Input: dimensioned drawing with shaded views. Units: mm. Origin: part minimum x, y, z. A direction names the side the tool comes from. Round coordinates to 2 decimals unless told otherwise and drop trailing zeros. Loops run counter-clockwise (first coordinate to the right, second up) from the corner with the lowest first, then second, coordinate; pieces in that order, holes last. Notation, with made-up numbers: (-4.75, 58) - (8.25, 58) arc R14 cw to (8.25, 74) - close; hole circle Ø6 at (-11.75, 54). An arc over 180 degrees is marked (long way). Answer as CSV lines item,"result".
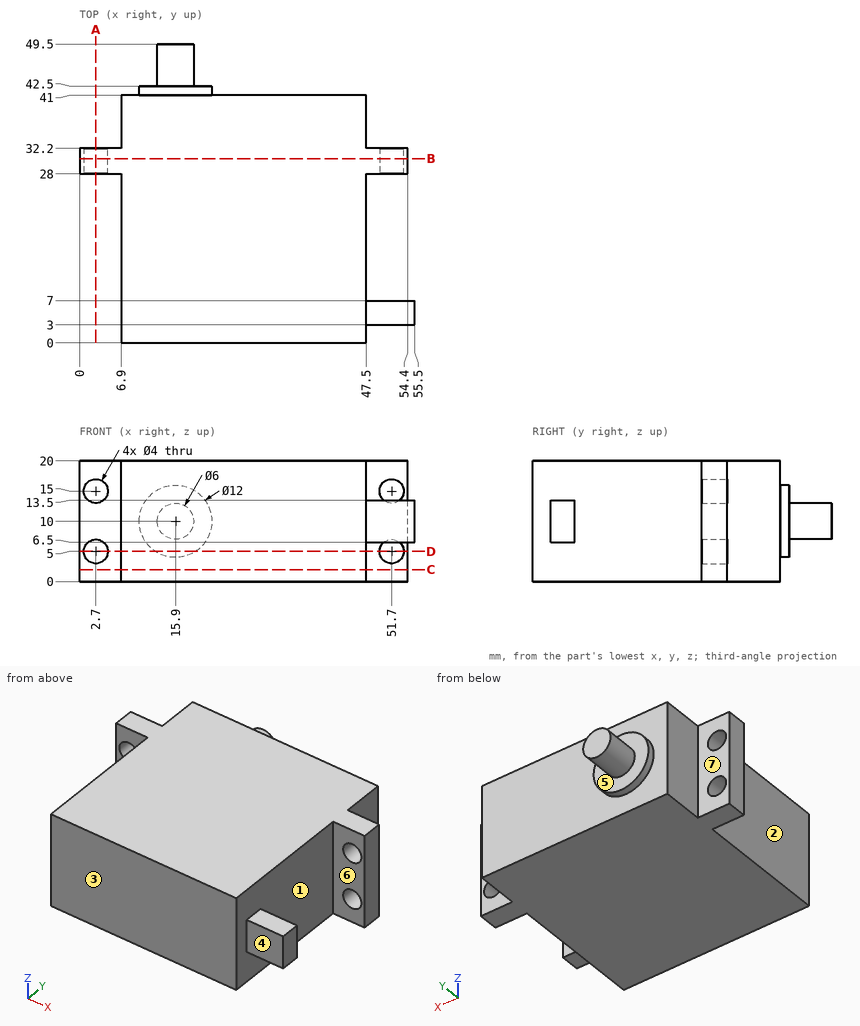
(1) Section A-A (x = 2.7). Output: boundary loops of the cut face in (y, z).
Findings below:
outline,"(28, 0) - (32.2, 0) - (32.2, 3) - (28, 3) - close; (28, 7) - (32.2, 7) - (32.2, 13) - (28, 13) - close; (28, 17) - (32.2, 17) - (32.2, 20) - (28, 20) - close"
(2) Draft query along Y for the marked faces 1, 2 and 3. Return one class per face: pulls with the +Y half, pulls with the -Y half, needs draft (parallel to the pull), parting line crosses it, or undercut.
Findings below:
face 1,"undercut"
face 2,"needs draft"
face 3,"pulls with the -Y half"
(3) Material intervals for line 1 along Z through (x, y) = (2.7, 29.7); line 2 along Z through (x, y) = (51, 29); line 3 along Y through (x, z) = (23, 13.25), sorted ascending.
Findings below:
line 1,"0 to 3, 7 to 13, 17 to 20"
line 2,"0 to 3.13, 6.87 to 13.13, 16.87 to 20"
line 3,"0 to 41"
(4) Section C-C (z = 2). Output: boundary loops of the cut face in (x, y).
Findings below:
outline,"(0, 28) - (6.9, 28) - (6.9, 0) - (47.5, 0) - (47.5, 28) - (54.4, 28) - (54.4, 32.2) - (47.5, 32.2) - (47.5, 41) - (6.9, 41) - (6.9, 32.2) - (0, 32.2) - close"
(5) Section D-D (z = 5). Output: boundary loops of the cut face in (x, y).
Findings below:
outline,"(0, 28) - (0.7, 28) - (0.7, 32.2) - (0, 32.2) - close; (4.7, 28) - (6.9, 28) - (6.9, 0) - (47.5, 0) - (47.5, 28) - (49.7, 28) - (49.7, 32.2) - (47.5, 32.2) - (47.5, 41) - (19.22, 41) - (19.22, 42.5) - (12.58, 42.5) - (12.58, 41) - (6.9, 41) - (6.9, 32.2) - (4.7, 32.2) - close; (53.7, 28) - (54.4, 28) - (54.4, 32.2) - (53.7, 32.2) - close"
(6) Pin query (flat end, axial travel): P1, Ø6, axis at y = 14.5, z = 7, coming from the +X side; P2, Ø1.2, axis at x = 52.5, y = 4.5, coming from the +Z side; P3, Ø2, axis at x = 51, z = 11, coming from the -Y side. Return the tip coordinate at first contact, or that it passes through.
Findings below:
P1,"x = 47.5"
P2,"z = 13.5"
P3,"y = 3"
(7) Section B-B (y = 30.5). Output: boundary loops of the cut face in (x, z).
Findings below:
outline,"(0, 0) - (54.4, 0) - (54.4, 20) - (0, 20) - close; hole circle Ø4 at (2.7, 5); hole circle Ø4 at (2.7, 15); hole circle Ø4 at (51.7, 5); hole circle Ø4 at (51.7, 15)"
(8) Access query for the marked faces 4, 5, 6 and 7. Directions: +Z, -Z, +X, -X, +Y, -Y. A direction counts if a zero-diameter tool reaches every point of the face in a straight line with its end or side. Return the directions, or none.
Findings below:
face 4,"+Z, -Z, +X, -Y"
face 5,"+Y"
face 6,"+Z, -Z, +X"
face 7,"+Z, -Z, -X, +Y"
